Check sheet for the modelled part. Datum: model origin and axes. Units: mm. A direction names the side the tool comes from. Round coordinates to 2 decimals unless told otherwise and drop trailing zeros. Order: outer loops, then holes, each group sorted by start corner. A loop starts at its lowest first (then second) coordinate and runs counter-clockwise, first axis right, second up.
from build123d import *

# Parameters (mm, degrees)
F1_DEPTH       = 127
F3_D           = 6.35
F3_CBORE_D     = 12.7
F3_CBORE_DEPTH = 6.35
F4_R           = 5.08
F5_W           = 32.5189703144
F5_H           = 77.4685703218
F6_DEPTH       = 65.1611467814
F7_R           = 5.08


with BuildPart() as f1:
    # F0 (on Front) → F1 (new body)
    with BuildSketch(Plane.XZ):
        Polygon((-60.8552582562, 38.7677326798), (-60.8552582562, 0), (17.7800003439, 0), (17.7800003439, 38.7677326798), (-29.5111350715, 57.6475299895), align=None)
    extrude(amount=F1_DEPTH)

    # F3 (through all)
    with Locations(Plane.XZ.offset(127)):
        with Locations((-21.01104334, 25.3676697612)):
            CounterBoreHole(F3_D / 2, F3_CBORE_D / 2, F3_CBORE_DEPTH)

    # F4
    f4_edges = [f1.edges().sort_by_distance(p)[0] for p in [
        (-21.537629, -127, 0),
        (17.78, -127, 19.383866),
        (17.78, -63.5, 0),
    ]]
    fillet(f4_edges, radius=F4_R)

    # F5 (on face) → F6 (cut, through all)
    with BuildSketch(Plane(origin=(15.7936314356, 0, 39.5607405457), x_dir=(0.9287247193, 0, -0.3707700038), z_dir=(0.3707700038, 0, 0.9287247193))):
        with Locations((-23.8889742177, -54.570266977)):
            Rectangle(F5_W, F5_H)
    extrude(amount=-F6_DEPTH, mode=Mode.SUBTRACT)

    # F7
    f7_edges = [f1.edges().sort_by_distance(p)[0] for p in [
        (-32.361451, -15.835982, 27.223292),
        (0.24646, -15.835982, 21.194763),
        (0.24646, -93.304552, 21.194763),
        (-32.361451, -93.304552, 27.223292),
    ]]
    fillet(f7_edges, radius=F7_R)


solid = f1.part
1) Scan lines: line 1 (Y direction, x = -6, z = 20.5); line 2 (Y direction, x = 6.5, z = 5); line 3 (Y direction, x = -34.5, z = 15.5). Record each from-to range of solid material in increasing order.
2) Sectioned sample at A-A on y = -85. Record the cut outline in (x, z), and give its area (3 significant figures).
3) Draft check along Z on faces 1 (the face through (-22, 0, 29)), 2 (the face through (-44.96, -62.61, 48.34)), 3 (the face through (-21.838, -123.869, 31.664)). Enter one of: pulls with the +Z half, pulls with the -Z half, needs draft (parallel to the pull), parting line crosses it, or undercut.
4) Gauge pin test, flat ends, axial feed: pin 1 (12 mm diameter, centred on x = -38.5, y = -69, fed in from +Z); pin 2 (7.5 mm diameter, centred on x = -21.01, z = 25.37, fed in from +Y); pin 3 (7.5 mm diameter, centred on x = -21.01, z = 25.37, fed in from -Y). Record the tip position at first contact, or that the pin passes through.
5) Sectioned sample at B-B on x = -55. Record the cut outline in (y, z).
6) Set-up check for faces 4 (the face through (-17, -15.836, 23)), 5 (the face through (-1.672, -91.856, 20.509)), 6 (the face through (-32.21, -55.04, 27.6)), 7 (the face through (-17.84, -7.81, 25.51)): record each of +Z, -Z, +X, -X, +Y, -Y from which the full face is reachable in a straight line by a thin tool's end or side.
Values found:
1. line 1: y = -127 to -93.3, -15.84 to 0
1. line 2: y = -127 to 0
1. line 3: y = -127 to -92.52, -16.63 to 0
2. outline: (-60.86, 0) - (-43.23, 0) - (-21.49, 54.45) - (-29.51, 57.65) - (-60.86, 38.77) - close; (-8.22, 0) - (12.7, 0) arc R5.08 ccw to (17.78, 5.08) - (17.78, 38.77) - (8.71, 42.39) - close
2. area: 2,090 mm2
3. face 1: needs draft
3. face 2: pulls with the +Z half
3. face 3: undercut
4. pin 1: stops at z = 55.85
4. pin 2: stops at y = 0
4. pin 3: stops at y = -120.65
5. outline: (-127, 5.08) arc R5.08 ccw to (-121.92, 0) - (0, 0) - (0, 42.29) - (-127, 42.29) - close
6. face 4: none
6. face 5: +Z
6. face 6: -Z
6. face 7: +Y, -Y
